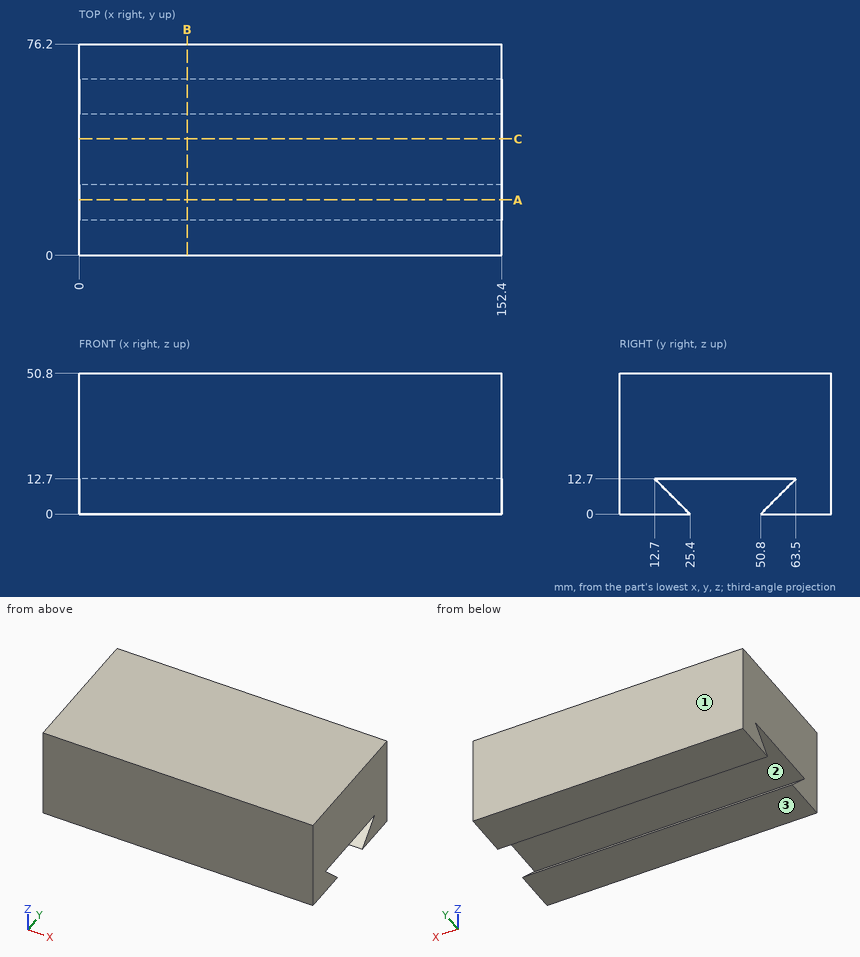
Check sheet for the drawn part. Datum: minimum x, y, z corner. Units: mm. Give positions to 0.01 mm unless a question says otherwise; leave off trailing zeros. Write each loop counter-clockwise with the first axis right and the second up, starting at its lowest first coordinate (ties: lowest second). Pieces come first, ordered by that corner, then holes. Notation, with made-up numbers: (9.25, 28.5) - (23.25, 28.5) arc R11 cw to (23.25, 43.5) - close; hole circle Ø6 at (58.5, -7.75). An arc over 180 degrees is marked (long way). Put each result on its own line as item: value.
1. Sectioned sample at C-C, the plane y = 42. Enter the section's corners in (x, z).
Ans:
outline: (0, 12.7) - (152.4, 12.7) - (152.4, 50.8) - (0, 50.8) - close
2. Sectioned sample at A-A, the plane y = 20. Enter the section's corners in (x, z), plus the area to 3 significant figures.
Ans:
outline: (0, 0) - (152.4, 0) - (152.4, 5.4) - (0, 5.4) - close; (0, 12.7) - (152.4, 12.7) - (152.4, 50.8) - (0, 50.8) - close
area: 6,630 mm²
3. Go/stop test with flat-tipped pins: pin 1 (6 mm diameter, centred on x = 39, y = 35.5, fed in from -Z); pin 2 (3 mm diameter, centred on y = 16, z = 9.5, fed in from +X). Record where each tip stops, or that it passes through.
Ans:
pin 1: stops at z = 12.7
pin 2: stops at x = 152.4
4. Draft check along Y on the marked faces 1, 2 and 3. Enter one of: +Y half, -Y half, draft (parallel to the pull), parting line (faces both ways), or undercut.
Ans:
face 1: +Y half
face 2: undercut
face 3: draft
5. Thickness scan on line 1 (Z direction, x = 136.5, y = 43); line 2 (Y direction, x = 41, z = 4); line 3 (Z direction, x = 58.5, y = 22.5). Record the ranges inside material, lowest first.
Ans:
line 1: z = 12.7 to 50.8
line 2: y = 0 to 21.4, 54.8 to 76.2
line 3: z = 0 to 2.9, 12.7 to 50.8
6. Sectioned sample at B-B, the plane x = 39. Enter the section's corners in (y, z), plus the area to 3 significant figures.
Ans:
outline: (0, 0) - (25.4, 0) - (12.7, 12.7) - (63.5, 12.7) - (50.8, 0) - (76.2, 0) - (76.2, 50.8) - (0, 50.8) - close
area: 3,390 mm²
